Input: part model. Units: mm. Frame: model coordinates. A direction names the side the tool comes from. Round coordinates to 2 decimals unless told otherwise and drop trailing zeros. Loops run counter-clockwise (first coordinate to the right, second up) from the corner with the lowest first, then second, coordinate; pieces in that order, holes last. Notation, with made-up numbers: (-12, -38) -> (0, -38) arc R12 ccw to (0, -25) -> close; hole circle Ø2 at (6.5, 19). An arc over 180 degrees is marked (long way). Answer in a Markdown table with one row per item. Add a question column.
Q1. Reachability of faces 1 (the face through (0, 19, 12)), 2 (the face through (-42.5, 0, 32)), 3 (the face through (29, 23, 20)), 4 (the face through (18, -10, 24.5)) from +Z, -Z, +X, -X, +Y, -Y: full face, straight path, thin tool, end or side. Return the list, or none.
Q2. Section D-D, the plane x = -34.5. Output: boundary loops of the cut face in (y, z).
Q3. Ray query, L1, parallel to X at y = -30, z = 32; L2, parallel to X at y = -16, z = 5; L3, parallel to X at y = -14, z = 8. Return the intervals inside material, ascending. Write a range as from..to.
Q4. Section B-B, the plane z = 15. Output: boundary loops of the cut face in (x, y).
Q5. Section A-A, the plane y = -21. Output: boundary loops of the cut face in (x, z).
Q6. Section C-C, the plane y = -27.5. Give the number of separate pieces and of enclosed holes in the cut face, and give its area (3 significant figures).
Q7. Mould query, pull axis Y, two halves, no side actions, for faces 5 (the face through (-0.66, 16.61, 15.46)), 6 (the face through (40, -21, 6)). Classes: pulls with the +Y half, pulls with the -Y half, needs draft (parallel to the pull), parting line crosses it, or undercut.
Q8. Pin query (flat end, axial travel): pin 1 (16.5 mm diameter, centred on y = -2, z = 28.5, fed in from -X); pin 2 (16.5 mm diameter, centred on y = 6, z = 25.5, fed in from +X); pin 3 (1.5 mm diameter, centred on x = 12.5, z = 16, fed in from -Y); pin 4 (1.8 mm diameter, centred on y = 27.5, z = 15, fed in from -X). Return the tip coordinate at first contact, or that it passes through.
```python
from build123d import *

# Parameters (mm, degrees)
ESQUISSE1_W              = 95
ESQUISSE1_H              = 65
BOSS_EXTRU_1_DEPTH       = 40
ESQUISSE3_R              = 40
ENL_V_MAT_EXTRU_1_DEPTH  = 12
ESQUISSE5_W              = 5
ESQUISSE5_H              = 20
ENL_V_MAT_EXTRU_2_DEPTH  = 90.895772982
ESQUISSE6_W              = 5
ESQUISSE6_H              = 20
ENL_V_MAT_EXTRU_3_DEPTH  = 90.895772982
ESQUISSE7_W              = 80
ESQUISSE7_H              = 22.5
ENL_V_MAT_EXTRU_4_DEPTH  = 12
ESQUISSE8_W              = 95
ESQUISSE8_H              = 12.5
ENL_V_MAT_EXTRU_5_DEPTH  = 45
ESQUISSE10_W             = 30
ESQUISSE10_H             = 65
ENL_V_MAT_EXTRU_6_DEPTH  = 17
ESQUISSE11_W             = 13.5
ESQUISSE11_H             = 15
ENL_V_MAT_EXTRU_7_DEPTH  = 90.895772982
ESQUISSE12_W             = 13.5
ESQUISSE12_H             = 15
ENL_V_MAT_EXTRU_8_DEPTH  = 90.895772982
ESQUISSE14_R             = 1
ENL_V_MAT_EXTRU_9_DEPTH  = 109.079831606
ESQUISSE15_R             = 1.25
ENL_V_MAT_EXTRU_10_DEPTH = 71.089228844
ESQUISSE16_R             = 1.25
ENL_V_MAT_EXTRU_11_DEPTH = 90.895772982


with BuildPart() as part:
    # Esquisse1 → Boss.-Extru.1 (new body)
    with BuildSketch(Plane.XY):
        Rectangle(ESQUISSE1_W, ESQUISSE1_H)
    extrude(amount=BOSS_EXTRU_1_DEPTH)

    # Esquisse3 → Enlèv. mat.-Extru.1 (cut)
    with BuildSketch(Plane(origin=(0, 0, 0), x_dir=(-1, 0, 0), z_dir=(0, 0, -1))):
        with Locations((0, -10)):
            Circle(ESQUISSE3_R)
    extrude(amount=-ENL_V_MAT_EXTRU_1_DEPTH, mode=Mode.SUBTRACT)

    # Esquisse5 → Enlèv. mat.-Extru.2 (cut, through all)
    with BuildSketch(Plane(origin=(0, 32.5, 0), x_dir=(1, 0, 0), z_dir=(0, 1, 0))):
        with Locations((-45, -30)):
            Rectangle(ESQUISSE5_W, ESQUISSE5_H)
    extrude(amount=-ENL_V_MAT_EXTRU_2_DEPTH, mode=Mode.SUBTRACT)

    # Esquisse6 → Enlèv. mat.-Extru.3 (cut, through all)
    with BuildSketch(Plane(origin=(0, 32.5, 0), x_dir=(1, 0, 0), z_dir=(0, 1, 0))):
        with Locations((45, -30)):
            Rectangle(ESQUISSE6_W, ESQUISSE6_H)
    extrude(amount=-ENL_V_MAT_EXTRU_3_DEPTH, mode=Mode.SUBTRACT)

    # Esquisse7 → Enlèv. mat.-Extru.4 (cut)
    with BuildSketch(Plane(origin=(0, 0, 0), x_dir=(-1, 0, 0), z_dir=(0, 0, -1))):
        with Locations((0, -21.25)):
            Rectangle(ESQUISSE7_W, ESQUISSE7_H)
    extrude(amount=-ENL_V_MAT_EXTRU_4_DEPTH, mode=Mode.SUBTRACT)

    # Esquisse8 → Enlèv. mat.-Extru.5 (cut)
    with BuildSketch(Plane.XZ.offset(32.5)):
        with Locations((0, 18.25)):
            Rectangle(ESQUISSE8_W, ESQUISSE8_H)
    extrude(amount=-ENL_V_MAT_EXTRU_5_DEPTH, mode=Mode.SUBTRACT)

    # Esquisse10 → Enlèv. mat.-Extru.6 (cut)
    with BuildSketch(Plane.XY.offset(40)):
        Rectangle(ESQUISSE10_W, ESQUISSE10_H)
    extrude(amount=-ENL_V_MAT_EXTRU_6_DEPTH, mode=Mode.SUBTRACT)

    # Esquisse11 → Enlèv. mat.-Extru.7 (cut, through all)
    with BuildSketch(Plane(origin=(0, 32.5, 0), x_dir=(1, 0, 0), z_dir=(0, 1, 0))):
        with Locations((-28.75, -27.5)):
            Rectangle(ESQUISSE11_W, ESQUISSE11_H)
    extrude(amount=-ENL_V_MAT_EXTRU_7_DEPTH, mode=Mode.SUBTRACT)

    # Esquisse12 → Enlèv. mat.-Extru.8 (cut, through all)
    with BuildSketch(Plane(origin=(0, 32.5, 0), x_dir=(1, 0, 0), z_dir=(0, 1, 0))):
        with Locations((28.75, -27.5)):
            Rectangle(ESQUISSE12_W, ESQUISSE12_H)
    extrude(amount=-ENL_V_MAT_EXTRU_8_DEPTH, mode=Mode.SUBTRACT)

    # Esquisse14 → Enlèv. mat.-Extru.9 (cut, through all)
    with BuildSketch(Plane.ZY.offset(47.5)):
        with Locations((15, 27.5)):
            Circle(ESQUISSE14_R)
        with Locations((15, 17.5)):
            Circle(ESQUISSE14_R)
    extrude(amount=-ENL_V_MAT_EXTRU_9_DEPTH, mode=Mode.SUBTRACT)

    # Esquisse15 → Enlèv. mat.-Extru.10 (cut, through all)
    with BuildSketch(Plane.XY.offset(40)):
        with Locations((-37.5, 22.5)):
            Circle(ESQUISSE15_R)
        with Locations((37.5, 22.5)):
            Circle(ESQUISSE15_R)
        with Locations((-37.5, -27.5)):
            Circle(ESQUISSE15_R)
        with Locations((37.5, -27.5)):
            Circle(ESQUISSE15_R)
    extrude(amount=-ENL_V_MAT_EXTRU_10_DEPTH, mode=Mode.SUBTRACT)

    # Esquisse16 → Enlèv. mat.-Extru.11 (cut, through all)
    with BuildSketch(Plane.XZ.offset(32.5)):
        with Locations(Location((42.5, 5, 0), (0, 0, 270))):
            Circle(ESQUISSE16_R)
        with Locations(Location((-42.5, 5, 0), (0, 0, 270))):
            Circle(ESQUISSE16_R)
    extrude(amount=-ENL_V_MAT_EXTRU_11_DEPTH, mode=Mode.SUBTRACT)


solid = part.part
```
Answer block:
| question | item | result |
|---|---|---|
| 1 | face 1 | -Z, -Y |
| 1 | face 2 | +Z, -X, +Y, -Y |
| 1 | face 3 | +Y, -Y |
| 1 | face 4 | -Z, +X, -X, -Y |
| 2 | outline | (-32.5, 35) -> (32.5, 35) -> (32.5, 40) -> (-32.5, 40) -> close; (10.24, 0) -> (32.5, 0) -> (32.5, 20) -> (12.5, 20) -> (12.5, 12) -> (10.24, 12) -> close; hole circle Ø2 at (17.5, 15); hole circle Ø2 at (27.5, 15) |
| 3 | L1 | -42.5..-35.5, -22..-15, 15..22, 35.5..42.5 |
| 3 | L2 | -47.5..-43.75, -41.25..-40, 40..41.25, 43.75..47.5 |
| 3 | L3 | -47.5..-40, 40..47.5 |
| 4 | outline | (-47.5, 12.5) -> (47.5, 12.5) -> (47.5, 16.5) -> (-47.5, 16.5) -> close; (-47.5, 18.5) -> (47.5, 18.5) -> (47.5, 26.5) -> (-47.5, 26.5) -> close; (-47.5, 28.5) -> (47.5, 28.5) -> (47.5, 32.5) -> (-47.5, 32.5) -> close; hole circle Ø2.5 at (-37.5, 22.5); hole circle Ø2.5 at (37.5, 22.5) |
| 5 | outline | (-47.5, 0) -> (-40, 0) -> (-40, 12) -> (-47.5, 12) -> close; (-42.5, 24.5) -> (-35.5, 24.5) -> (-35.5, 35) -> (-22, 35) -> (-22, 24.5) -> (-15, 24.5) -> (-15, 40) -> (-42.5, 40) -> close; (15, 24.5) -> (22, 24.5) -> (22, 35) -> (35.5, 35) -> (35.5, 24.5) -> (42.5, 24.5) -> (42.5, 40) -> (15, 40) -> close; (40, 0) -> (47.5, 0) -> (47.5, 12) -> (40, 12) -> close; hole circle Ø2.5 at (-42.5, 5); hole circle Ø2.5 at (42.5, 5) |
| 6 | separate pieces | 6 |
| 6 | enclosed holes | 2 |
| 6 | area | 662 mm^2 |
| 7 | face 5 | undercut |
| 7 | face 6 | needs draft |
| 8 | pin 1 | x = -42.5 |
| 8 | pin 2 | x = 42.5 |
| 8 | pin 3 | y = 12.5 |
| 8 | pin 4 | through |
